from build123d import *

# Parameters (mm, degrees)
VYSUNOUT1_DEPTH          = 8
SKICA2_R                 = 3
VYSUNOUT2_DEPTH          = 31
M3_Z_VITOV_D_RY1_D       = 3
ZKOSIT1_SIZE             = 1
SKICA5_W                 = 10.533076429
SKICA5_H                 = 13.637336759
ODEBRAT_VYSUNUT_M1_DEPTH = 2
ODEBRAT_VYSUNUT_M2_DEPTH = 2
SKICA7_W                 = 10.597302505
SKICA7_H                 = 5.566259902
ODEBRAT_VYSUNUT_M3_DEPTH = 5
ZAOBLIT1_R               = 4
SKICA8_R                 = 0.875
ODEBRAT_VYSUNUT_M4_DEPTH = 6
LINPOLE1_COUNT           = 6
LINPOLE1_PITCH           = 4
LINPOLE1_COUNT_DIR2      = 4
LINPOLE1_PITCH_DIR2      = 50


with BuildPart() as part:
    # Skica1 → Vysunout1 (new body)
    with BuildSketch(Plane.XY):
        with BuildLine():
            Line((0, 0), (10, 0))
            ThreePointArc((10, 0), (15, -5), (10, -10))
            Line((10, -10), (0, -10))
            ThreePointArc((0, -10), (-5, -5), (0, 0))
        make_face()
    extrude(amount=VYSUNOUT1_DEPTH)

    # Skica2 → Vysunout2 (add)
    with BuildSketch(Plane.XY.offset(8)):
        with Locations((0, -5)):
            Circle(SKICA2_R)
    extrude(amount=VYSUNOUT2_DEPTH)

    # M3 závitové díry1 (through all)
    with Locations(Plane.XY.offset(8)):
        with Locations((10, -5)):
            Hole(M3_Z_VITOV_D_RY1_D / 2)

    # Zkosit1
    zkosit1_edges = [part.edges().sort_by_distance(p)[0] for p in [
        (-3, -5, 8),
    ]]
    chamfer(zkosit1_edges, length=ZKOSIT1_SIZE)

    # Skica5 → Odebrat vysunutím1 (cut)
    with BuildSketch(Plane(origin=(0, 0, 0), x_dir=(-1, 0, 0), z_dir=(0, 0, -1))):
        with Locations((-11.266538215, -4.925069579)):
            Rectangle(SKICA5_W, SKICA5_H)
    extrude(amount=-ODEBRAT_VYSUNUT_M1_DEPTH, mode=Mode.SUBTRACT)

    # Skica6 → Odebrat vysunutím2 (cut)
    with BuildSketch(Plane(origin=(0, 0, 2), x_dir=(-1, 0, 0), z_dir=(0, 0, -1))):
        with BuildLine():
            Line((-6, -1), (-6, -9))
            Line((-6, -9), (-10, -9))
            ThreePointArc((-10, -9), (-14, -5), (-10, -1))
            Line((-10, -1), (-6, -1))
        make_face()
    extrude(amount=-ODEBRAT_VYSUNUT_M2_DEPTH, mode=Mode.SUBTRACT)

    # Skica7 → Odebrat vysunutím3 (cut)
    with BuildSketch(Plane(origin=(0, 0, 0), x_dir=(-1, 0, 0), z_dir=(0, 0, -1))):
        with Locations((0.298651253, -1.716870049)):
            Rectangle(SKICA7_W, SKICA7_H)
        with Locations((0.298651253, -8.283129951)):
            Rectangle(SKICA7_W, SKICA7_H)
    extrude(amount=-ODEBRAT_VYSUNUT_M3_DEPTH, mode=Mode.SUBTRACT)

    # Zaoblit1
    zaoblit1_edges = [part.edges().sort_by_distance(p)[0] for p in [
        (-5, -5, 0),
    ]]
    fillet(zaoblit1_edges, radius=ZAOBLIT1_R)

    # Skica8 → Odebrat vysunutím4 (cut)
    with BuildSketch(Plane(origin=(0, -8, 0), x_dir=(-1, 0, 0), z_dir=(0, 1, 0))):
        with Locations(Location((0, 36, 0), (0, 0, 270))):  # turned: the seam where the file's is
            Circle(SKICA8_R)
    odebrat_vysunut_m4 = extrude(amount=ODEBRAT_VYSUNUT_M4_DEPTH, mode=Mode.SUBTRACT)

    # LinPole1: Odebrat vysunut_m4 6 × 4
    with Locations(*[Vector(0, 0, -1) * (i * LINPOLE1_PITCH) + Vector(0, 0, -1) * (j * LINPOLE1_PITCH_DIR2) for i in range(LINPOLE1_COUNT) for j in range(LINPOLE1_COUNT_DIR2) if (i, j) != (0, 0)]):
        add(odebrat_vysunut_m4, mode=Mode.SUBTRACT)


solid = part.part
Check sheet for the modelled part. Datum: model origin and axes. Units: mm. A direction names the side the tool comes from. Coordinates: 2 decimals unless noted, no trailing zeros. Write each loop counter-clockwise with the first axis right and the second up, starting at its lowest first coordinate (ties: lowest second). Pieces come first, ordered by that corner, then holes.
Item 1: Depth check by flat-ended pin: pin 1 Ø1.4 at (x, z) = (0, 32) entering from -Y; pin 2 Ø5 at (y, z) = (-4, 31.5) entering from +X; pin 3 Ø2 at (y, z) = (-2.5, 2.5) entering from -X; pin 4 Ø1.3 at (x, y) = (-2.5, -2.5) entering from -Z. Enter the tip coordinate at first touch or a pass-through.
Numbers:
pin 1: passes through
pin 2: stops at x = 3
pin 3: stops at x = 5
pin 4: stops at z = 5
Item 2: Cross-section at C-C on y = -2.75. Count the separate pieces of the cut face and the enclosed holes in it, then the cut area to 3 significant figures.
Numbers:
separate pieces: 1
enclosed holes: 6
area: 183 mm2
Item 3: Cross-section at B-B on z = 13.5. Record the boundary of the cut face in (x, y).
Numbers:
outline: circle Ø6 at (0, -5)
Item 4: Access from +Z, -Z, +X, -X, +Y, -Y to the whole of each face (thin tool, end or side, straight path). Record for faces 1 (the face through (0, -2, 5)), 2 (the face through (2.86, -4.1, 23.79)), 3 (the face through (8, -9, 3)), 4 (the face through (5, -8, 2)).
Numbers:
face 1: -Z, -X, +Y
face 2: +Z
face 3: -Z
face 4: -Z, -X, -Y
Item 5: Cross-section at A-A on z = 4.5. Record the boundary of the cut face in (x, y), then the cut area to 3 significant figures.
Numbers:
outline: (-4.97, -5.5) - (5, -5.5) - (5, -10) - (10, -10) arc R5 ccw to (10, 0) - (5, 0) - (5, -4.5) - (-4.97, -4.5) arc R5 ccw to start; hole circle Ø3 at (10, -5)
area: 92.2 mm2
Item 6: Mould release check, pull along X, two halves, no side actions. Record for faces 5 (the face through (-5, -5, 6)), 6 (the face through (0, -5.5, 2)), 7 (the face through (14, -5, 3)): released by +X, released by -X, zero draft, split by the parting line, or undercut.
Numbers:
face 5: released by -X
face 6: zero draft
face 7: undercut
Item 7: Scan lines: probe 1 along Z at (x, y) = (2.5, -8.5); probe 2 along X at (y, z) = (-4, 16) (3 decimals); probe 3 along X at (y, z) = (-5.75, 16) (3 decimals). Record each from-to range of solid material in increasing order.
Numbers:
probe 1: z = 5 to 8
probe 2: x = -2.828 to -0.875, 0.875 to 2.828
probe 3: x = -2.905 to -0.875, 0.875 to 2.905
